```python
from build123d import *

# Parameters (mm, degrees)
SKETCH1_W           = 65.6
SKETCH1_H           = 29
SKETCH1_R           = 2.5
BOSS_EXTRUDE1_DEPTH = 10
BOSS_EXTRUDE2_DEPTH = 7.5
CIRPATTERN1_COUNT   = 4


with BuildPart() as part:
    # Sketch1 → Boss-Extrude1 (new body)
    with BuildSketch(Plane(origin=(0, 0, 0), x_dir=(1, 0, 0), z_dir=(0, 1, 0))):
        Rectangle(SKETCH1_W, SKETCH1_H)
        with Locations((-19.85, 10)):
            Circle(SKETCH1_R, mode=Mode.SUBTRACT)
        with Locations((19.85, 10)):
            Circle(SKETCH1_R, mode=Mode.SUBTRACT)
        with Locations((19.85, -10)):
            Circle(SKETCH1_R, mode=Mode.SUBTRACT)
        with Locations((-19.85, -10)):
            Circle(SKETCH1_R, mode=Mode.SUBTRACT)
    extrude(amount=BOSS_EXTRUDE1_DEPTH)

    # Sketch2 → Boss-Extrude2 (add)
    with BuildSketch(Plane(origin=(0, 10, 0), x_dir=(1, 0, 0), z_dir=(0, 1, 0))):
        Polygon((-10, 5.5), (-10, -5.5), (-7.7, -3.2), (-7.7, -5), (-6.06, -5), (-3.9, -2.84), (-3.9, 2.84), (-6.06, 5), (-7.7, 5), (-7.7, 3.2), align=None)
    boss_extrude2 = extrude(amount=BOSS_EXTRUDE2_DEPTH)

    # CirPattern1: Boss-Extrude2 ×4 about axis
    cirpattern1_axis = Axis((0, 0, 0), (0, 1, 0))
    for i in range(1, CIRPATTERN1_COUNT):
        add(boss_extrude2.rotate(cirpattern1_axis, i * 360 / CIRPATTERN1_COUNT))


solid = part.part
```
Could you check a few things on this model? Use its own coordinates, in mm. A direction names the side the tool comes from. Coordinates: 2 decimals unless noted, no trailing zeros. Write each loop counter-clockwise with the first axis right and the second up, starting at its lowest first coordinate (ties: lowest second). Pieces come first, ordered by that corner, then holes. Notation, with made-up numbers: (-16, -10.75) -> (31, -10.75) arc R16 cw to (31, 2.25) -> close; hole circle Ø4 at (48, 36.25). An arc over 180 degrees is marked (long way). Write item = value, one per line. Start each with the question number.
(1) I need wall thicknesses on line 1 (Z direction, x = -19.85, y = 3); line 2 (X direction, y = 3.25, z = -10); line 3 (X direction, y = 14.25, z = 1). Which ranges of each line are inside material? Lowest first, please. Write a range as [from, to].
(2) Which directions (+Z, -Z, +X, -X, +Y, -Y) give clear straight access to the entire face, cutting with the end or side of a thin tool? Please do faces 1 (the face through (0, 14, 10)), 2 (the face through (10, 14, 0)), 3 (the face through (-7, 14, -5)), 4 (the face through (0, 14, 3.9)).
(3) We'd pull the mould along X, two halves only. Please class faces 5 (the face through (7, 14, -5)), 6 (the face through (-10, 14, 0)), 7 (the face through (5, 14, 7)): released by +X, released by -X, zero draft, split by the parting line, or undercut.
(4) I want a section at A-A (x = -19.85). Please give me the cut outline in (y, z), plus the area to 3 significant figures.
(5) I want a section at C-C (y = 2.75). Please give me the cut outline in (x, z).
(6) I want a section at B-B (z = -1). Please give me the cut outline in (x, y).
(7) Will these pins go through, and if not, where does the flat tip stop? pin 1 (4 mm diameter, centred on x = 19.85, z = -10, fed in from -Y); pin 2 (3 mm diameter, centred on y = 14.5, z = 0.5, fed in from -X); pin 3 (4.5 mm diameter, centred on x = -0.5, y = 14, fed in from +Z); pin 4 (2 mm diameter, centred on y = 13.5, z = -2.5, fed in from +X).
(8) I want a section at D-D (z = 11). Please give me the cut outline in (x, y).
Result set:
q1.line_1 = [-14.5, -12.5], [-7.5, 7.5], [12.5, 14.5]
q1.line_2 = [-32.8, -22.35], [-17.35, 17.35], [22.35, 32.8]
q1.line_3 = [-10, -3.9], [3.9, 10]
q2.face_1 = +Z, +X, -X, +Y
q2.face_2 = +Z, -Z, +X, +Y
q2.face_3 = -Z, +Y
q2.face_4 = +Y
q3.face_5 = undercut
q3.face_6 = released by -X
q3.face_7 = released by +X
q4.outline = (0, -14.5) -> (10, -14.5) -> (10, -12.5) -> (0, -12.5) -> close; (0, -7.5) -> (10, -7.5) -> (10, 7.5) -> (0, 7.5) -> close; (0, 12.5) -> (10, 12.5) -> (10, 14.5) -> (0, 14.5) -> close
q4.area = 190 mm2
q5.outline = (-32.8, -14.5) -> (32.8, -14.5) -> (32.8, 14.5) -> (-32.8, 14.5) -> close; hole circle Ø5 at (-19.85, -10); hole circle Ø5 at (-19.85, 10); hole circle Ø5 at (19.85, -10); hole circle Ø5 at (19.85, 10)
q6.outline = (-32.8, 0) -> (32.8, 0) -> (32.8, 10) -> (10, 10) -> (10, 17.5) -> (3.9, 17.5) -> (3.9, 10) -> (-3.9, 10) -> (-3.9, 17.5) -> (-10, 17.5) -> (-10, 10) -> (-32.8, 10) -> close
q7.pin_1 = through
q7.pin_2 = -10
q7.pin_3 = 10
q7.pin_4 = 10
q8.outline = (-32.8, 0) -> (-22.14, 0) -> (-22.14, 10) -> (-32.8, 10) -> close; (-17.56, 0) -> (17.56, 0) -> (17.56, 10) -> (-17.56, 10) -> close; (22.14, 0) -> (32.8, 0) -> (32.8, 10) -> (22.14, 10) -> close
